Answer from the drawing. Dimensions are ordinates in mm from the lowest x, y and z of the part. A direction names the side the tool comes from. Round coordinates to 2 decimals unless told otherwise and drop trailing zeros. Loops run counter-clockwise (first coordinate to the right, second up) from the corner with the lowest first, then second, coordinate; pieces in that order, holes last. Notation, with made-up numbers: (53.5, 20) -> (83.5, 20) arc R14 cw to (83.5, 28) -> close; hole circle Ø11 at (71, -18). An arc over 180 degrees is marked (long way). One line per question, with ' | ' between items.
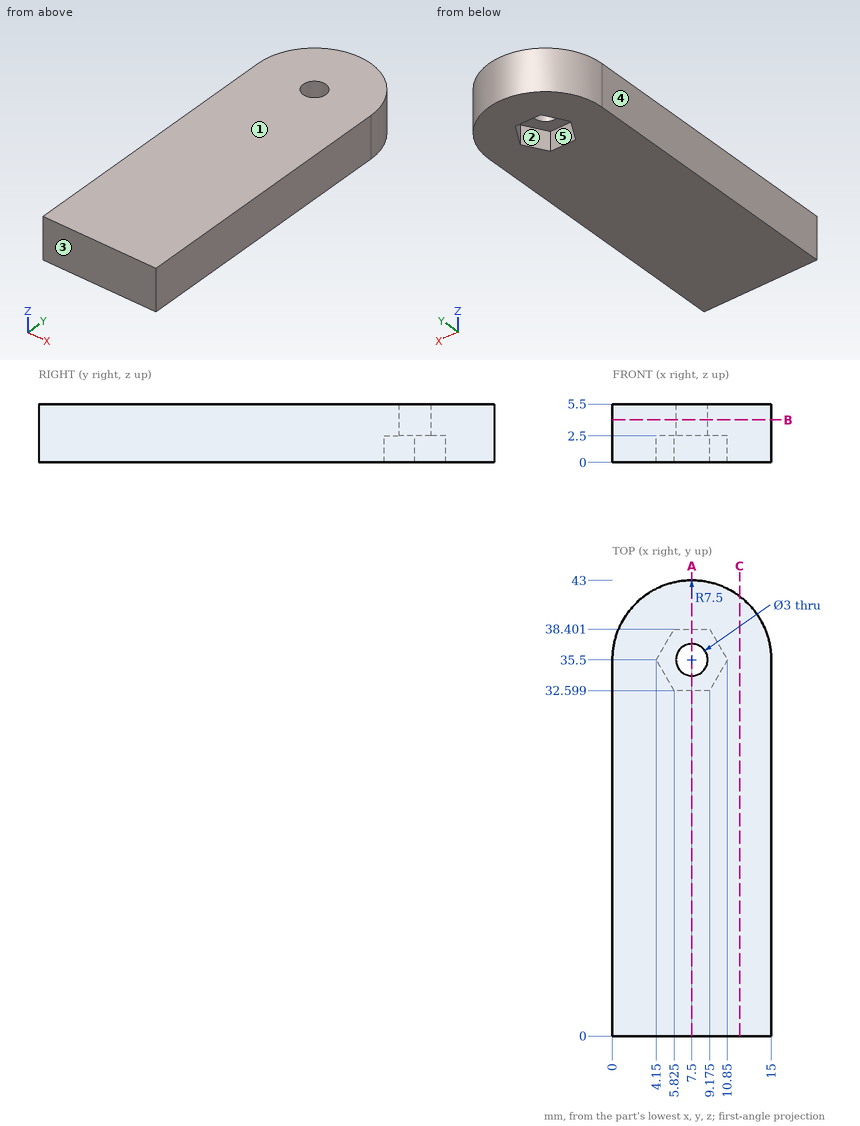
Q1. Given pin 1 Ø1.7 at (x, y) = (6.5, 36.5) entering from -Z; pin 2 Ø1.5 at (x, z) = (7, 3) entering from +Y; pin 3 Ø2 at (x, z) = (11, 0.5) entering from +Y, each flat-ended and moving along its own axis, determine where each tip first touches the part or whether it passes through.
Numbers:
pin 1: z = 2.5 | pin 2: y = 43 | pin 3: y = 42.57
Q2. A cutting plane is placed at B-B on z = 4. Give the vertices of the cut face in (x, y).
Numbers:
outline: (0, 0) -> (15, 0) -> (15, 35.5) arc R7.5 ccw to (0, 35.5) -> close; hole circle Ø3 at (7.5, 35.5)
Q3. A cutting plane is placed at A-A on x = 7.5. Give the vertices of the cut face in (y, z).
Numbers:
outline: (0, 0) -> (32.6, 0) -> (32.6, 2.5) -> (34, 2.5) -> (34, 5.5) -> (0, 5.5) -> close; (37, 2.5) -> (38.4, 2.5) -> (38.4, 0) -> (43, 0) -> (43, 5.5) -> (37, 5.5) -> close
Q4. Find the intervals of material crossed by line 1 (Y direction, x = 7.5, z = 3.65); line 2 (X direction, y = 36.5, z = 5.05); line 3 (Y direction, x = 8.5, z = 0.55), in increasing order. Write a range as from..to.
Numbers:
line 1: 0..34, 37..43 | line 2: 0.07..6.38, 8.62..14.93 | line 3: 0..32.6, 38.4..42.93
Q5. A cutting plane is placed at C-C on x = 12. Give the vertices of the cut face in (y, z).
Numbers:
outline: (0, 0) -> (41.5, 0) -> (41.5, 5.5) -> (0, 5.5) -> close
Q6. For a pull along Y with two mould halves and no side action, classify the marked faces 3, 4 and 5 as pulls with the +Y half, pulls with the -Y half, needs draft (parallel to the pull), parting line crosses it, or undercut.
Numbers:
face 3: pulls with the -Y half | face 4: needs draft | face 5: undercut
Q7. For the marked faces 1 and 2, determine the directions among +Z, -Z, +X, -X, +Y, -Y from which every point of the face is accessible in a straight line to the end or side of a thin tool.
Numbers:
face 1: +Z, +X, -X, +Y, -Y | face 2: -Z
